Can you work these out from the model? Positions are in its coordinate system, mm. A direction names the side the tool comes from. Round coordinates to 2 decimals unless told otherwise and drop trailing zeros. Loops run counter-clockwise (first coordinate to the right, second up) from the corner with the lowest first, then second, coordinate; pieces in that order, holes last. Notation, with made-up numbers: (36, -23.5) -> (73, -23.5) arc R23 cw to (73, -2.5) -> close; hole circle Ø4 at (-21, -36). An arc over 180 degrees is marked (long way). Write item = value, one per line.
from build123d import *

# Parameters (mm, degrees)
SKETCH1_R           = 6
BOSS_EXTRUDE1_DEPTH = 7
BOSS_EXTRUDE2_DEPTH = 4


with BuildPart() as part:
    # Sketch1 → Boss-Extrude1 (new body)
    with BuildSketch(Plane.XY):
        with BuildLine():
            Line((17.517837099, -9.650149397), (-17.517837099, -9.650149397))
            ThreePointArc((-17.517837099, -9.650149397), (0, 20), (17.517837099, -9.650149397))
        make_face()
        with Locations((0, 8.349850603)):
            Circle(SKETCH1_R, mode=Mode.SUBTRACT)
    extrude(amount=BOSS_EXTRUDE1_DEPTH)

    # Sketch5 → Boss-Extrude2 (add)
    with BuildSketch(Plane.XZ.offset(9.650149397)):
        Polygon((-24.517837099, -4), (-24.517837099, 0), (-17.517837099, 0), (-17.517837099, 7), (-24.517837099, 7), (-24.517837099, 11), (-39.517837099, 11), (-39.517837099, -4), align=None)
        Polygon((24.517837099, -4), (39.517837099, -4), (39.517837099, 11), (24.517837099, 11), (24.517837099, 7), (17.517837099, 7), (17.517837099, 0), (24.517837099, 0), align=None)
    extrude(amount=-BOSS_EXTRUDE2_DEPTH)


solid = part.part
1. We'd pull the mould along Y, two halves only. Please class faces 1 (the flat face through (-1, -9.65, 4)), 2 (the cylindrical face through (-0.52, 19.993, 3.451)), 3 (the flat face through (-24.518, -8, 9)), 4 (the cylindrical face through (-4.422, 12.405, 3.451)): released by +Y, released by -Y, zero draft, split by the parting line, or undercut.
Entries:
face_1 = released by -Y
face_2 = undercut
face_3 = zero draft
face_4 = undercut
2. Suppose I cut it at B-B, the plane x = 0. List the corners of the cut face in (y, z) for me, and give its area (3 significant figures).
Entries:
outline = (-9.65, 0) -> (2.35, 0) -> (2.35, 7) -> (-9.65, 7) -> close; (14.35, 0) -> (20, 0) -> (20, 7) -> (14.35, 7) -> close
area = 124 mm²
3. Suppose I cut it at C-C, the plane z = 2. List the corners of the cut face in (x, y) for me, and give its area (3 significant figures).
Entries:
outline = (-39.52, -9.65) -> (39.52, -9.65) -> (39.52, -5.65) -> (19.19, -5.65) arc R20 ccw (long way) to (-19.19, -5.65) -> (-39.52, -5.65) -> close; hole circle Ø12 at (0, 8.35)
area = 1,050 mm²
4. Suppose I cut it at A-A, the plane z = -2.5. List the corners of the cut face in (x, y) for me.
Entries:
outline = (-39.52, -9.65) -> (-24.52, -9.65) -> (-24.52, -5.65) -> (-39.52, -5.65) -> close; (24.52, -9.65) -> (39.52, -9.65) -> (39.52, -5.65) -> (24.52, -5.65) -> close
5. I need wall thicknesses on line 1 (Z direction, x = 14, y = -7.75); line 2 (Y direction, x = -25, z = 4.75); line 3 (Y direction, x = 5, z = 1.5). Which ranges of each line are inside material? Lowest first, please. Write a range as [from, to].
Entries:
line_1 = [0, 7]
line_2 = [-9.65, -5.65]
line_3 = [-9.65, 5.03], [11.67, 19.36]
6. Suppose I cut it at D-D, the plane y = 0. List the corners of the cut face in (x, z) for me, and give its area (3 significant figures).
Entries:
outline = (-20, 0) -> (20, 0) -> (20, 7) -> (-20, 7) -> close
area = 280 mm²
7. For faces 5 (the flat face through (0, 2, 7)), 6 (the flat face through (-24.518, -8, -2)), 7 (the flat face through (32, -8, 11)), which set-ups out of +Z, -Z, +X, -X, +Y, -Y let a thin tool reach every point of the face, with its end or its side?
Entries:
face_5 = +Z, +Y, -Y
face_6 = -Z, +Y, -Y
face_7 = +Z, +X, -X, +Y, -Y
8. I'm going to push flat-ended pins straight in: pin 1 (7.5 mm diameter, centred on x = 27, z = 5.5, fed in from +Y); pin 2 (2 mm diameter, centred on x = 5, y = 16.5, fed in from -Z); pin 3 (2 mm diameter, centred on y = 0.5, z = 1.5, fed in from -X). Where does each tip first touch, or does it pass through?
Entries:
pin_1 = -5.65
pin_2 = 0
pin_3 = -20
